Autodesk Inventor part; units mm, degrees
ref_plane "Work Plane1" through (0, 0, 1.5875) normal (0, 0, -1) x (-1, 0, 0)
ref_plane "Work Plane2" through (0, 0, 130.683) normal (0, 0, -1) x (-1, 0, 0)
ref_plane "Work Plane3" through (0, 0, 160.3375) normal (0, 0, 1) x (1, 0, 0)
sketch "Sketch1" plane through (0, 0, 0) normal (0, 0, 1) x (1, 0, 0)
  arc A0 (-1, 4.6563) -> (1, 4.6563) centre (0, 0) ccw
  line L0 (-1, 3.7625) -> (1, 3.7625)
  line L1 (1, 3.7625) -> (1, 4.6563)
  line L2 (1, 5.7625) -> (-1, 5.7625) construction
  line L3 (-1, 5.7625) -> (-1, 4.6563) construction
  arc A1 (1, 4.6563) -> (-1, 4.6563) centre (0, 0) ccw construction
  line L4 (-1, 4.6563) -> (-1, 3.7625)
  line L5 (1, 4.6563) -> (1, 5.7625) construction
  dimension "d0" = 9.525
  dimension "d3" = 2
  dimension "d4" = 2
  dimension "d5" = 1
  dimension "d6" = 3.7625
extrude "Extrusion1" add sketch "Sketch1" along normal blind 161.925
ref_plane "Work Plane1" through (0, 0, 1.5875) normal (0, 0, -1) x (-1, 0, 0)
sketch "Sketch2" plane through (0, 0, 1.5875) normal (0, 0, -1) x (-1, 0, 0)
  line L0 (-1, 3.7625) -> (-1, 4.6563)
  line L1 (1, 3.7625) -> (-1, 3.7625)
  line L2 (1, 4.6563) -> (1, 3.7625)
  arc A0 (-1, 4.6563) -> (1, 4.6563) centre (0, 0) ccw
  arc A1 (-1, 3.8735) -> (1, 3.8735) centre (0, 0) ccw
  arc A2 (1, 3.8735) -> (-1, 3.8735) centre (0, 0) ccw construction
  dimension "d9" = 0.762
extrude "Extrusion2" cut sketch "Sketch2" against normal blind 0.762 contours A1 L2 A0 L0
ref_plane "Work Plane2" through (0, 0, 130.683) normal (0, 0, -1) x (-1, 0, 0)
sketch "Sketch3" plane through (0, 0, 130.683) normal (0, 0, -1) x (-1, 0, 0)
  arc A0 (-1, 3.8735) -> (1, 3.8735) centre (0, 0) ccw
  line L0 (-1, 3.7625) -> (-1, 4.6563)
  arc A1 (-1, 4.6563) -> (1, 4.6563) centre (0, 0) ccw
  line L1 (1, 4.6563) -> (1, 3.7625)
  line L2 (1, 3.7625) -> (-1, 3.7625)
extrude "Extrusion3" cut sketch "Sketch3" against normal blind 0.762 contours A0 L1 A1 L0
ref_plane "Work Plane3" through (0, 0, 160.3375) normal (0, 0, 1) x (1, 0, 0)
sketch "Sketch4" plane through (0, 0, 160.3375) normal (0, 0, 1) x (1, 0, 0)
  arc A0 (-1, 3.8735) -> (1, 3.8735) centre (0, 0) ccw
  line L0 (-1, 3.7625) -> (1, 3.7625)
  line L1 (-1, 4.6563) -> (-1, 3.7625)
  line L2 (1, 3.7625) -> (1, 4.6563)
  arc A1 (-1, 4.6563) -> (1, 4.6563) centre (0, 0) ccw
extrude "Extrusion4" cut sketch "Sketch4" against normal blind 1.016 contours A0 L2 A1 L1
equation "\"d4\" = d3"
properties part number "vertical drive shaft 2"
Geometry check sheet. Reference: the model listing, model coordinates, mm. A direction names the side the tool comes from. Give positions to 0.01 mm unless a question says otherwise; leave off trailing zeros. Write each loop counter-clockwise with the first axis right and the second up, starting at its lowest first coordinate (ties: lowest second). Pieces come first, ordered by that corner, then holes. Notation, with made-up numbers: (-36, -4) - (-10, -4) arc R17 cw to (-10, 19) - close; hole circle Ø10 at (-30, -32). An arc over 180 degrees is marked (long way). Use a Markdown table: item, result.
Q1. Thickness scan on L1, parallel to Z at x = -1.5, y = 4 (1 decimal); L2, parallel to X at y = 4, z = 8.5; L3, parallel to X at y = 0.5, z = 152.5. Record the ranges inside material, lowest first. Write a range as [from, to].
Computed:
| item | result |
|---|---|
| L1 | z = [0, 1.6], [2.3, 130.7], [131.4, 159.3], [160.3, 161.9] |
| L2 | x = [-2.58, -1], [1, 2.58] |
| L3 | x = [-4.74, 4.74] |
Q2. Go/stop test with flat-tipped pins: P1, Ø1, axis at y = 4.5, z = 60.5, coming from the -X side; P2, Ø1.6, axis at x = 0, z = 60.5, coming from the +Y side; P3, Ø4.5, axis at x = 1.5, y = 1, coming from the -Z side; P4, Ø1, axis at x = 2, z = 93.5, coming from the -Y side. Record where each tip stops, or that it passes through.
Computed:
| item | result |
|---|---|
| P1 | stops at x = -2.58 |
| P2 | stops at y = 3.76 |
| P3 | stops at z = 0 |
| P4 | stops at y = -4.52 |
Q3. Section check A-A, the plane y = -2. Enter the section's corners in (x, z) (1 decimal), then the cut area to 3 significant figures.
Computed:
| item | result |
|---|---|
| outline | (-4.3, 0) - (4.3, 0) - (4.3, 1.6) - (3.5, 1.6) - (3.5, 2.3) - (4.3, 2.3) - (4.3, 130.7) - (3.5, 130.7) - (3.5, 131.4) - (4.3, 131.4) - (4.3, 159.3) - (3.5, 159.3) - (3.5, 160.3) - (4.3, 160.3) - (4.3, 161.9) - (-4.3, 161.9) - (-4.3, 160.3) - (-3.5, 160.3) - (-3.5, 159.3) - (-4.3, 159.3) - (-4.3, 131.4) - (-3.5, 131.4) - (-3.5, 130.7) - (-4.3, 130.7) - (-4.3, 2.3) - (-3.5, 2.3) - (-3.5, 1.6) - (-4.3, 1.6) - close |
| area | 1,400 mm² |
Q4. Section check C-C, the plane z = 23. Enter the section's corners in (x, y).
Computed:
| item | result |
|---|---|
| outline | (-1, 3.76) - (-1, 4.66) arc R4.76 ccw (long way) to (1, 4.66) - (1, 3.76) - close |
Q5. Set-up check for faces 4 (the face through (3, -3, 131.445)), 5 (the face through (0.2, -4.76, 65.62)): record each of +Z, -Z, +X, -X, +Y, -Y from which the full face is reachable in a straight line by a thin tool's end or side.
Computed:
| item | result |
|---|---|
| face 4 | none |
| face 5 | +Z, -Z |
Q6. Section check B-B, the plane x = -2.5. Enter the section's corners in (y, z) (1 decimal), then the cut area to 3 significant figures.
Computed:
| item | result |
|---|---|
| outline | (-4.1, 0) - (4.1, 0) - (4.1, 1.6) - (3.1, 1.6) - (3.1, 2.3) - (4.1, 2.3) - (4.1, 130.7) - (3.1, 130.7) - (3.1, 131.4) - (4.1, 131.4) - (4.1, 159.3) - (3.1, 159.3) - (3.1, 160.3) - (4.1, 160.3) - (4.1, 161.9) - (-4.1, 161.9) - (-4.1, 160.3) - (-3.1, 160.3) - (-3.1, 159.3) - (-4.1, 159.3) - (-4.1, 131.4) - (-3.1, 131.4) - (-3.1, 130.7) - (-4.1, 130.7) - (-4.1, 2.3) - (-3.1, 2.3) - (-3.1, 1.6) - (-4.1, 1.6) - close |
| area | 1,310 mm² |
Q7. Draft check along Z on faces 1 (the face through (0.2, -4.76, 0.78)), 2 (the face through (-3, -3, 159.322)), 3 (the face through (0, 0, 0)). Enter one of: pulls with the +Z half, pulls with the -Z half, needs draft (parallel to the pull), parting line crosses it, or undercut.
Computed:
| item | result |
|---|---|
| face 1 | needs draft |
| face 2 | undercut |
| face 3 | pulls with the -Z half |
